```python
from build123d import *

# Parameters (mm, degrees)
F0_W     = 2
F0_H     = 70
F1_DEPTH = 25


with BuildPart() as f1:
    # F0 (on Front) → F1 (new body)
    with BuildSketch(Plane.XZ):
        Polygon((-127.978955, 72), (-127.978955, 0), (-21.978955, 0), (-21.978955, 2), (-23.978955, 2), (-73.978955, 2), (-73.978955, 72), (-75.978955, 72), (-75.978955, 2), (-125.978955, 2), (-125.978955, 72), align=None)
        with Locations((-22.978955, 37)):
            Rectangle(F0_W, F0_H)
    extrude(amount=F1_DEPTH)


solid = f1.part
```
The model under review builds one solid part; all positions refer to its coordinate system, in mm. A direction names the side the tool comes from. Give positions to 0.01 mm unless a question says otherwise; leave off trailing zeros. Write each loop counter-clockwise with the first axis right and the second up, starting at its lowest first coordinate (ties: lowest second). Pieces come first, ordered by that corner, then holes. Notation, with made-up numbers: M 70.5,-3 L 106.5,-3 A15 ccw 106.5,5 Z; hole C 19,-21.75 d6. An arc over 180 degrees is marked long. Write item = value, one per line. Start each with the question number.
Q1. Machinability: for faces 1 (the face through (-101, -12, 2)), 2 (the face through (-75, 0, 26)), which of the approach directions +Z, -Z, +X, -X, +Y, -Y give a long, thin tool a straight path to every point of the face, cutting with its end or side? Answer none if there is none.
Q2. For line 1 (X direction, y = -5.75, z = 44.5); line 2 (Z direction, x = -33.5, y = -10.5), list the stretches that pass through material, from the lowest coordinate up.
Q3. We need section C-C (x = -85). State the section outline as (y, z) points, plus the area to 3 significant figures.
Q4. Clearance check with a flat-ended pin moving along its axis: pin 1 (1 mm diameter, centred on x = -83.5, y = -11.5, fed in from +Z). State where the tip first meets the part, or that it passes through.
Q5. Mouldability with a two-part tool opening along X and no side actions: class faces 3 (the face through (-125.979, -12, 37)), 4 (the face through (-21.979, -12, 35)), 5 (the face through (-75, -25, 26)) as released by +X, released by -X, zero draft, split by the parting line, or undercut.
Q6. We need section A-A (z = 41.5). State the section outline as (x, y) points.
Q7. We need section B-B (y = -20). State the section outline as (x, z) points, plus the area to 3 significant figures.
Result set:
q1.face_1 = +Z, +Y, -Y
q1.face_2 = +Z, -Z, +X, -X, +Y
q2.line_1 = -127.98 to -125.98, -75.98 to -73.98, -23.98 to -21.98
q2.line_2 = 0 to 2
q3.outline = M -25,0 L 0,0 L 0,2 L -25,2 Z
q3.area = 50.0 mm2
q4.pin_1 = 2
q5.face_3 = undercut
q5.face_4 = released by +X
q5.face_5 = zero draft
q6.outline = M -127.98,-25 L -125.98,-25 L -125.98,0 L -127.98,0 Z; M -75.98,-25 L -73.98,-25 L -73.98,0 L -75.98,0 Z; M -23.98,-25 L -21.98,-25 L -21.98,0 L -23.98,0 Z
q7.outline = M -127.98,0 L -21.98,0 L -21.98,72 L -23.98,72 L -23.98,2 L -73.98,2 L -73.98,72 L -75.98,72 L -75.98,2 L -125.98,2 L -125.98,72 L -127.98,72 Z
q7.area = 632 mm2
